```python
from build123d import *

# Parameters (mm, degrees)
BOSS_EXTRUDE1_DEPTH = 3
FILLET1_R           = 0.6
BOSS_EXTRUDE2_DEPTH = 1


with BuildPart() as part:
    # Sketch1 → Boss-Extrude1 (new body)
    with BuildSketch(Plane.XY):
        with BuildLine():
            Line((2.813726101, -7.233722886), (2.813726101, 6.312465104))
            add(Edge.make_bspline(
                [(2.813726101, 6.312465104), (2.504718004, 6.264404648), (1.893497156, 6.064800789), (0.890081325, 5.34240891), (-0.080852226, 3.898834313), (-0.647319625, 2.07334315), (-0.882193889, 0.581865897), (-0.93021587, -0.107691535), (-0.938912211, -0.460628891)],
                knots=[0.032675075, 0.032675075, 0.032675075, 0.032675075, 0.153501113, 0.274327151, 0.515979228, 0.757631304, 0.878457343, 0.999283381, 0.999283381, 0.999283381, 0.999283381], degree=3))
            add(Edge.make_bspline(
                [(-0.938912211, -0.460628891), (-0.93021587, -0.813566247), (-0.882193889, -1.503123679), (-0.647319625, -2.994600932), (-0.080852226, -4.820092095), (0.890081325, -6.263666692), (1.893497156, -6.986058571), (2.504718004, -7.18566243), (2.813726101, -7.233722886)],
                knots=[0.032675075, 0.032675075, 0.032675075, 0.032675075, 0.153501113, 0.274327151, 0.515979228, 0.757631304, 0.878457343, 0.999283381, 0.999283381, 0.999283381, 0.999283381], degree=3))
        make_face()
    extrude(amount=BOSS_EXTRUDE1_DEPTH)

    # Fillet1
    fillet1_edges = [part.edges().sort_by_distance(p)[0] for p in [
        (2.813726101, -7.233722886, 1.5),
        (2.813726101, 6.312465104, 1.5),
    ]]
    fillet(fillet1_edges, radius=FILLET1_R)

    # Sketch3 → Boss-Extrude2 (add)
    with BuildSketch(Plane.XY.offset(3)):
        with BuildLine():
            Line((3.613726101, -6.42120663), (3.613726101, 5.499948848))
            ThreePointArc((3.613726101, 5.499948848), (2.954184531, 6.688107639), (1.596981367, 6.756780552))
            add(Edge.make_bspline(
                [(1.596981367, 6.756780552), (1.282061762, 6.602245138), (0.994843741, 6.407135645), (0.467503364, 5.947936377), (0.233787218, 5.690400118), (-0.184066224, 5.140618178), (-0.370152574, 4.845270148), (-0.699300989, 4.232833375), (-0.841194277, 3.918340305), (-1.089857286, 3.276540027), (-1.196610753, 2.94922689), (-1.38071085, 2.283872115), (-1.458163179, 1.944713712), (-1.648747035, 0.922143409), (-1.722037558, 0.234076304), (-1.739155024, -0.460628891)],
                knots=[0, 0, 0, 0, 0.125, 0.125, 0.25, 0.25, 0.375, 0.375, 0.5, 0.5, 0.625, 0.625, 0.75, 0.75, 1, 1, 1, 1], degree=3))
            add(Edge.make_bspline(
                [(-1.739155024, -0.460628891), (-1.722036272, -1.15538629), (-1.648742974, -1.84324583), (-1.458332057, -2.865153843), (-1.380793827, -3.204774963), (-1.196784843, -3.869910467), (-0.98366247, -4.523264457), (-0.70170709, -5.148763327), (-0.375964944, -5.756542709), (-0.189209114, -6.054473312), (0.231167863, -6.608835903), (0.46405952, -6.865638613), (0.858736471, -7.210145529), (0.998171212, -7.317980735), (1.288068017, -7.512889958), (1.439226487, -7.600625828), (1.596981367, -7.678038334)],
                knots=[0, 0, 0, 0, 0.25, 0.25, 0.375, 0.375, 0.5, 0.625, 0.625, 0.75, 0.75, 0.875, 0.875, 0.9375, 0.9375, 1, 1, 1, 1], degree=3))
            ThreePointArc((1.596981367, -7.678038334), (2.954184531, -7.609365421), (3.613726101, -6.42120663))
        make_face()
    extrude(amount=BOSS_EXTRUDE2_DEPTH)


solid = part.part
```
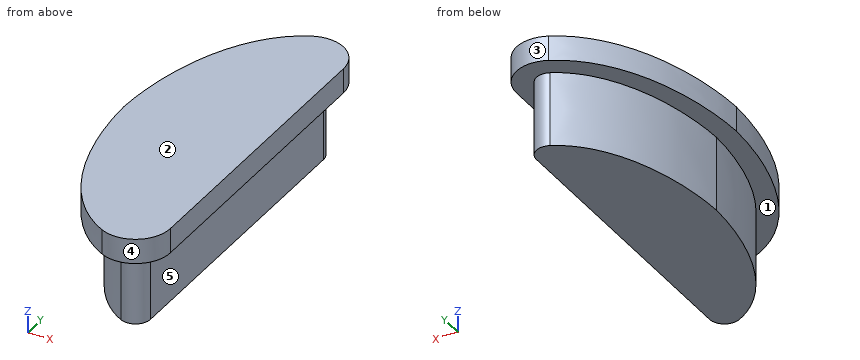
Check sheet for the modelled part. Datum: model origin and axes. Units: mm. Face numbers are marked on the shaded views. A direction names the side the tool comes from. Coordinates: 2 decimals unless noted, no trailing zeros. Write item = value, one per line. Start each with the question number.
1. Mould release check, pull along Y, two halves, no side actions. Record for the marked faces 3, 4 and 5: pulls with the +Y half, pulls with the -Y half, needs draft (parallel to the pull), parting line crosses it, or undercut.
2. Go/stop test with a flat-tipped pin: pin 1 (1.5 mm diameter, centred on y = 2, z = 2, fed in from +X). Record where the tip stops, or that it passes through.
3. Tool access check on the marked faces 1 and 2. Record the directions out of +Z, -Z, +X, -X, +Y, -Y that give a thin tool (end or side, any length) a straight path to the whole face; none if there is none.
4. Thickness scan on probe 1 along Z at (x, y) = (-1.05, -2.75); probe 2 along X at (y, z) = (4.25, 1.9); probe 3 along Y at (x, z) = (1.55, 1). Record the ranges inside material, lowest first.
The answers:
q1.face_3 = pulls with the +Y half
q1.face_4 = pulls with the -Y half
q1.face_5 = needs draft
q2.pin_1 = 2.81
q3.face_1 = -Z
q3.face_2 = +Z, +X, -X, +Y, -Y
q4.probe_1 = 3 to 4
q4.probe_2 = 0.22 to 2.81
q4.probe_3 = -6.72 to 5.8
